Autodesk Inventor part; units mm, degrees
ref_plane "YZ Plane" through (0, 0, 0) normal (1, 0, 0) x (0, 1, 0)
ref_plane "XZ Plane" through (0, 0, 0) normal (0, 1, 0) x (-1, 0, 0)
ref_plane "XY Plane" through (0, 0, 0) normal (0, 0, 1) x (1, 0, 0)
sketch "Sketch3" plane through (0, 0, 0) normal (0, 1, 0) x (-1, 0, 0)
  circle A0 centre (0, 0) radius 62.5
  dimension "d10" = 125
extrude "Extrusion3" add sketch "Sketch3" along normal blind 15
sketch "Sketch9" plane through (0, 0, 0) normal (0, -1, 0) x (1, 0, 0)
  circle A0 centre (0, 0) radius 50
  circle A1 centre (-50, 0) radius 4
  circle A2 centre (-25, -43.3013) radius 4
  circle A3 centre (25, -43.3013) radius 4
  circle A4 centre (50, 0) radius 4
  circle A5 centre (25, 43.3013) radius 4
  circle A6 centre (-25, 43.3013) radius 4
  dimension "d45" = 100
  dimension "d46" = 8
  dimension "d49" = 360
extrude "Extrusion8" cut sketch "Sketch9" against normal blind 20 contours A0 A4 | A0 A4 | A5 A0 | A0 A5 | A3 A0 | A0 A3 | A6 A0 | A0 A6 | A2 A0 | A0 A2 | A1 A0 | A0 A1
sketch "Sketch10" plane through (0, 15, 0) normal (0, 1, 0) x (1, 0, 0)
  circle A0 centre (25, 43.3013) radius 4
  circle A1 centre (0, 0) radius 50
  circle A2 centre (0, 50) radius 4
  circle A3 centre (0, 0) radius 31.5
  dimension "d53" = 8
  dimension "d54" = 63
extrude "Extrusion9" add sketch "Sketch10" along normal blind 9 contours A3
extrude "Extrusion10" add sketch "Sketch10" along normal blind 5 contours A2 A1 | A1 A2
ref_plane "Work Plane1" through (-20, 0, -20) normal (-1, 0, 0) x (0, 0, 1)
sketch "Sketch14" plane through (-20, 0, -20) normal (-1, 0, 0) x (0, 0, 1)
  line L0 (20, -1) -> (20, -74)
  arc A0 (20, -1) -> (19, 0) centre (19, -1) ccw
  line L1 (19, -75) -> (0, -75)
  arc A1 (19, -75) -> (20, -74) centre (19, -74) ccw
  line L2 (0, -85) -> (19, -85)
  arc A2 (19, -85) -> (30, -74) centre (19, -74) ccw
  line L3 (30, -74) -> (30, -5)
  line L4 (30, -5) -> (30, 0)
  line L5 (30, 0) -> (19, 0)
  line L6 (0, -75) -> (0, -85)
  point P0 (20, 0)
  point P1 (20, -75)
  dimension "d92" = 75
  dimension "d93" = 1
  dimension "d94" = 20
  dimension "d95" = 1
  dimension "d96" = 10
  dimension "d102" = 75
extrude "Extrusion16" add sketch "Sketch14" against normal blind 35
extrude "Extrusion17" cut sketch "Sketch14" against normal blind 5
fillet "Fillet4" radius 1 8 edges at (15, -80, -20) (-15, -80, -20) (-15, -81.7782, 6.7782) (-15, -85, -10.5) (-15, -37, 10) (15, -81.7782, 6.7782) (15, -37, 10) (15, -85, -10.5)
properties part number "EndEffector" material "Steel, High Strength, Low Alloy"
CAD build for the part. Positions are in the model's coordinates, mm. A direction names the side the tool comes from. Round coordinates to 2 decimals unless told otherwise and drop trailing zeros. Order: outer loops, then holes, each group sorted by start corner. A loop starts at its lowest first (then second) coordinate and runs counter-clockwise, first axis right, second up. Notation, with made-up numbers: (-5, -33.75) - (42, -33.75) arc R27 cw to (42, -11.75) - close; hole circle Ø10 at (55.5, -31). An arc over 180 degrees is marked (long way). Answer in a Markdown table with one row per item. Add a question column.
(1) Drop flat-ended pins along their axis: pin 1 Ø14 at (x, y) = (6, -47) entering from +Z; pin 2 Ø8 at (x, y) = (-16.5, 10.5) entering from +Z; pin 3 Ø5 at (x, z) = (-43, 26) entering from -Y. Give the stop position or say it passes through.
(2) Band-saw the part on B-B on x = 0. List the corners of the cut face in (y, z), and give its area (3 significant figures).
(3) Band-saw the part on C-C on z = 14. List the corners of the cut face in (x, y).
(4) Band-saw the part on D-D on y = -45.5. List the corners of the cut face in (x, z).
(5) Band-saw the part on A-A on x = -50. List the corners of the cut face in (y, z).
(6) 3-axis set-ups, long thin cutter, end or side, ignore diameter. For faces 1 (the face through (0, -75, -10)), 2 (the face through (15, -51, 1)), 3 (the face through (29, 15, 15)): which of +Z, -Z, +X, -X, +Y, -Y reach the whole face in a straight line?
(7) Mould opens along X. For faces 4 (the face through (21.8, 7.4, 40.9)), 5 (the face through (-4.101, 19.437, 31.232)), 6 (the face through (0, -80, -20)) say: +X half, -X half, draft (parallel to the pull), parting line (faces both ways), or undercut.
(8) Probe L1, parallel to Z at x = 25, y = 9; L2, parallel to X at y = -35.5, z = 1; L3, parallel to Y at x = 15.5, z = -52. List the from-to ranges inside material, lowest first. Write a range as [from, to].
Data:
| question | item | result |
|---|---|---|
| 1 | pin 1 | stops at z = 10 |
| 1 | pin 2 | stops at z = 61.24 |
| 1 | pin 3 | stops at y = 0 |
| 2 | outline | (-85, -20) - (-75, -20) - (-75, -1) arc R1 cw to (-74, 0) - (-1, 0) arc R1 cw to (0, -1) - (0, -62.5) - (15, -62.5) - (15, -54) - (20, -54) - (20, -46) - (15, -46) - (15, -31.5) - (24, -31.5) - (24, 31.5) - (15, 31.5) - (15, 62.5) - (0, 62.5) - (0, 10) - (-74, 10) arc R11 ccw to (-85, -1) - close |
| 2 | area | 3,510 mm^2 |
| 3 | outline | (-60.91, 0) - (60.91, 0) - (60.91, 15) - (28.22, 15) - (28.22, 24) - (-28.22, 24) - (-28.22, 15) - (-60.91, 15) - close |
| 4 | outline | (-15, 0) - (15, 0) - (15, 9) arc R1 ccw to (14, 10) - (-14, 10) arc R1 ccw to (-15, 9) - close |
| 5 | outline | (0, -37.5) - (15, -37.5) - (15, -4) - (0, -4) - close; (0, 4) - (15, 4) - (15, 37.5) - (0, 37.5) - close |
| 6 | face 1 | -Z, +X, -X |
| 6 | face 2 | +Z, -Z, +X, -Y |
| 6 | face 3 | +Y |
| 7 | face 4 | undercut |
| 7 | face 5 | parting line |
| 7 | face 6 | draft |
| 8 | L1 | z = [-57.28, -47.3], [-39.3, 39.3], [47.3, 57.28] |
| 8 | L2 | x = [-15, 15] |
| 8 | L3 | y = [0, 15] |
